from build123d import *

# Parameters (mm, degrees)
F0_W          = 177.8
F0_H          = 31.75
F5_DEPTH      = 22.225
F1_W          = 2.54
F1_H          = 2.54
F2_DEPTH      = 22.225
F2_DEPTH_BACK = 22.225
F3_R          = 3.81
F4_DEPTH      = 101.6


with BuildPart() as f5:
    # F0 (on Front) → F5 (new body, symmetric)
    with BuildSketch(Plane.XZ):
        Rectangle(F0_W, F0_H)
    extrude(amount=F5_DEPTH, both=True)

    # F1 (on Front) → F2 (cut, two sides)
    with BuildSketch(Plane.XZ) as f2_sk:
        with Locations((-65.0875, -14.605)):
            Rectangle(F1_W, F1_H)
        with Locations((46.0375, -14.605)):
            Rectangle(F1_W, F1_H)
    extrude(amount=F2_DEPTH, mode=Mode.SUBTRACT)
    extrude(f2_sk.sketch, amount=-F2_DEPTH_BACK, mode=Mode.SUBTRACT)

    # F3 (on face) → F4 (cut)
    with BuildSketch(Plane.XZ.offset(22.225)):
        with BuildLine():
            Line((-87.2850343585, -9.8690753803), (-88.9, -4.5820707456))
            add(Edge.make_bspline(
                [(-88.9, -4.5820707456), (-23.5271696001, 19.7381507605), (41.3550932653, 15.875), (88.9, 2.2290744901)],
                knots=[0, 0, 0, 0, 177.9304125197, 177.9304125197, 177.9304125197, 177.9304125197], degree=3))
            ThreePointArc((88.9, 2.2290744901), (74.4536678544, -2.1727649281), (68.10375, -15.875))
            Line((68.10375, -15.875), (90.8870175481, -24.3202205747))
            Line((90.8870175481, -24.3202205747), (97.0551893115, -13.2175106555))
            Line((97.0551893115, -13.2175106555), (95.2541902661, 10.2215418592))
            Line((95.2541902661, 10.2215418592), (84.6801921725, 31.5457955003))
            Line((84.6801921725, 31.5457955003), (-24.4083367288, 31.5457955003))
            Line((-24.4083367288, 31.5457955003), (-91.2008285522, 31.5457955003))
            Line((-91.2008285522, 31.5457955003), (-99.3075743318, -4.2296038009))
            Line((-99.3075743318, -4.2296038009), (-93.3156237006, -24.4964528829))
            Line((-93.3156237006, -24.4964528829), (-70.4052746296, -15.875))
            Line((-70.4052746296, -15.875), (-87.2850343585, -9.8690753803))
        make_face()
        with Locations((37.4968686472, 0.5141830338)):
            Circle(F3_R)
        with Locations((50.1968686472, 0.5141830338)):
            Circle(F3_R)
        with Locations((62.8967040475, 0.578842176)):
            Circle(F3_R)
        with BuildLine():
            Line((-8.0186231062, -30.1359239966), (37.8020815551, -15.875))
            ThreePointArc((37.8020815551, -15.875), (-7.4899233878, -4.7422597793), (-52.7819283307, -15.875))
            Line((-52.7819283307, -15.875), (-8.0186231062, -30.1359239966))
        make_face()
    extrude(amount=-F4_DEPTH, mode=Mode.SUBTRACT)


solid = f5.part
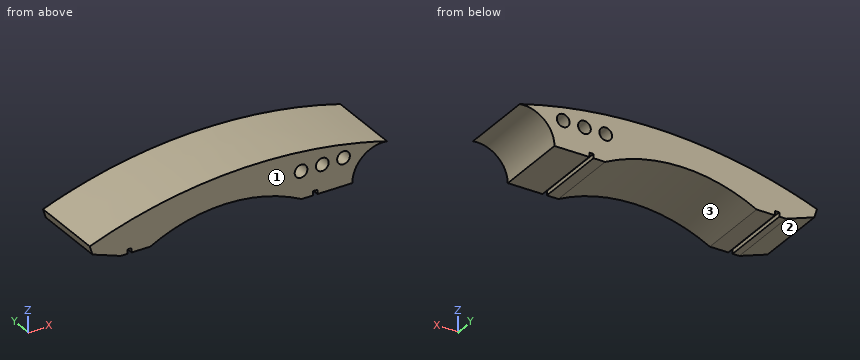
CAD build for the part. Positions are in the model's coordinates, mm. Face numbers are marked on the shaded views. Round coordinates to 2 decimals unless told otherwise and drop trailing zeros. Use one line per item in the form item = value.
Q1. Two-plate mould, pull along X, no slides. Class the marked faces 1, 2 and 3: +X half, -X half, draft (parallel to the pull), parting line (faces both ways), or undercut.
Recorded:
face_1 = draft
face_2 = -X half
face_3 = undercut
Q2. Saw through at A-A on y = -9.5. State how many separate pieces and enclosed holes the cut face has, then the cut area to 3 significant figures.
Recorded:
separate_pieces = 1
enclosed_holes = 3
area = 3,090 mm^2
Q3. Flat gauge pins, fed straight in: P1, Ø6, axis at y = -13, z = -9.5, coming from the +X side; P2, Ø12, axis at x = 62.9, z = 0.58, coming from the +Y side (3 decimals); P3, Ø6, axis at y = -5, z = -7.5, coming from the +X side; P4, Ø6, axis at x = -8.5, y = 16, coming from the +Z side. Where does each tip first touch, or does it go through?
Recorded:
P1 = 70.8
P2 = 22.225
P3 = 72.21
P4 = 12.66
Q4. Probe L1, parallel to Z at x = 62.5, y = 11 (3 decimals); L2, parallel to Z at x = 63, y = 20 (3 decimals); L3, parallel to Z at x = -43, y = 13.5. List the from-to ranges inside material, lowest first.
Recorded:
L1 = -15.875 to -3.21, 4.368 to 8.384
L2 = -15.875 to -3.23, 4.387 to 8.293
L3 = -11.42 to 8.15
